Job drawing, mm, ordinate dimensions from the low corner. One solid piece. Round coordinates to 2 decimals unless told otherwise and drop trailing zeros. Order: outer loops, then holes, each group sorted by start corner. A loop starts at its lowest first (then second) coordinate and runs counter-clockwise, first axis right, second up. Notation, with made-up numbers: (38.25, 9) -> (93.25, 9) arc R5 cw to (93.25, 15) -> close; hole circle Ø7 at (5, 5). An arc over 180 degrees is marked (long way). Use CSV: the item, a comma, the result in double quotes.
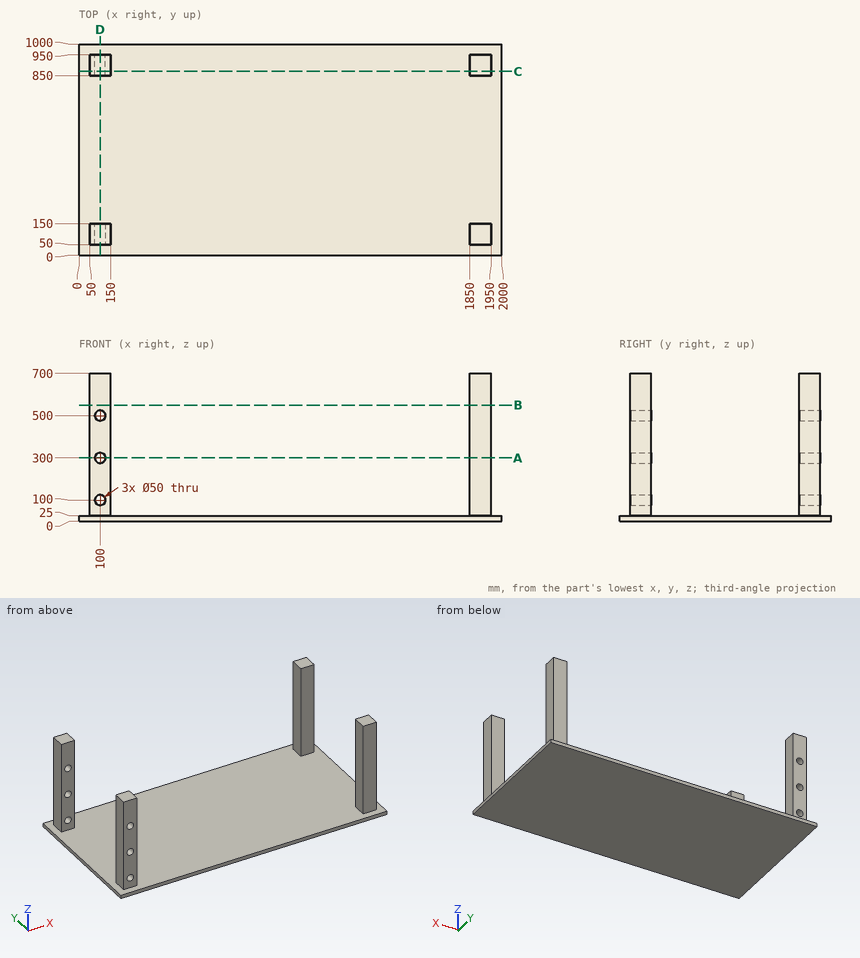
(1) Probe probe 1 along Z at (x, y) = (100, 126.5); probe 2 along X at (y, z) = (112, 500); probe 3 along X at (y, z) = (84, 264.5). List the from-to ranges inside material, lowest first. Write a range as [from, to].
Reply:
probe 1,"[0, 75], [125, 275], [325, 475], [525, 700]"
probe 2,"[50, 75], [125, 150], [1850, 1950]"
probe 3,"[50, 150], [1850, 1950]"
(2) Cut at D-D, the plane x = 100. State how many separate pieces and enclosed holes the cut face has, then the cut area to 3 significant figures.
Reply:
separate pieces,"7"
enclosed holes,"0"
area,"130,000 mm2"
(3) Drop a flat-ended pin along its axis: P1, Ø5, axis at x = 207.5, y = 568, coming from the +Z side. Give the stop position or say it passes through.
Reply:
P1,"z = 25"
(4) Cut at B-B, the plane z = 550. Give the cut face in (x, y).
Reply:
outline,"(50, 50) -> (150, 50) -> (150, 150) -> (50, 150) -> close; (50, 850) -> (150, 850) -> (150, 950) -> (50, 950) -> close; (1850, 50) -> (1950, 50) -> (1950, 150) -> (1850, 150) -> close; (1850, 850) -> (1950, 850) -> (1950, 950) -> (1850, 950) -> close"
(5) Cut at A-A, the plane z = 300. Give the cut face in (x, y), then the cut area to 3 significant figures.
Reply:
outline,"(50, 50) -> (75, 50) -> (75, 150) -> (50, 150) -> close; (50, 850) -> (75, 850) -> (75, 950) -> (50, 950) -> close; (125, 50) -> (150, 50) -> (150, 150) -> (125, 150) -> close; (125, 850) -> (150, 850) -> (150, 950) -> (125, 950) -> close; (1850, 50) -> (1950, 50) -> (1950, 150) -> (1850, 150) -> close; (1850, 850) -> (1950, 850) -> (1950, 950) -> (1850, 950) -> close"
area,"30,000 mm2"
(6) Cut at C-C, the plane y = 870.5. Give the cut face in (x, z), then the cut area to 3 significant figures.
Reply:
outline,"(0, 0) -> (2000, 0) -> (2000, 25) -> (1950, 25) -> (1950, 700) -> (1850, 700) -> (1850, 25) -> (150, 25) -> (150, 700) -> (50, 700) -> (50, 25) -> (0, 25) -> close; hole circle Ø50 at (100, 100); hole circle Ø50 at (100, 300); hole circle Ø50 at (100, 500)"
area,"179,000 mm2"
